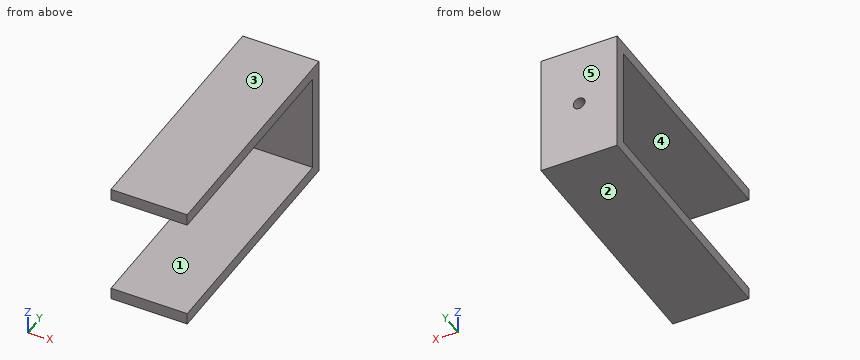
Autodesk Inventor part; units mm, degrees
ref_plane "YZ Plane" through (0, 0, 0) normal (1, 0, 0) x (0, 1, 0)
ref_plane "XZ Plane" through (0, 0, 0) normal (0, 1, 0) x (-1, 0, 0)
ref_plane "XY Plane" through (0, 0, 0) normal (0, 0, 1) x (1, 0, 0)
sketch "Boceto1" plane through (0, 0, 0) normal (0, 0, 1) x (1, 0, 0)
  line L0 (0, 0) -> (130, 0)
  line L1 (130, 0) -> (130, 420)
  line L2 (130, 420) -> (0, 420)
  line L3 (0, 420) -> (0, 0)
  circle A0 centre (65, 210) radius 10
  dimension "d0" = 130
  dimension "d1" = 420
  dimension "d2" = 130
  dimension "d10" = 20
extrude "Extrusión1" add sketch "Boceto1" along normal blind 210 contours L3 L2 L1 L0 | A0
sketch "Boceto2" plane through (130, 0, 0) normal (1, 0, 0) x (0, 0, -1)
  line L0 (-210, 420) -> (-210, 0)
  line L1 (-210, 0) -> (-190, 0)
  line L2 (0, 0) -> (-210, 0)
  line L3 (-190, 0) -> (-190, 400)
  line L4 (-190, 400) -> (-20, 400)
  line L5 (0, 420) -> (0, 0)
  line L6 (-20, 400) -> (-20, 0)
  line L7 (-20, 0) -> (0, 0)
  dimension "d5" = 20
  dimension "d6" = 400
  dimension "d7" = 170
extrude "Extrusión2" cut sketch "Boceto2" against normal blind 210
sketch "Boceto3" plane through (0, 420, 0) normal (0, 1, 0) x (1, 0, 0)
  line L0 (130, 0) -> (0, 0)
  line L1 (130, -210) -> (0, -210)
  line L2 (0, 0) -> (130, -210)
  line L3 (130, 0) -> (0, -210)
  circle A0 centre (65, -105) radius 10
  dimension "d11" = 20
hole "Agujero1" at (65, 420, 105) direction (0, -1, 0) diameter 20 end through all
properties part number "Soporteguia"
The listing builds one solid part. Answer for the finished solid, in the listing's coordinates (mm). Face numbers are marked on the shaded views. A direction names the side the tool comes from. Coordinates: 2 decimals unless noted, no trailing zeros. Loops run counter-clockwise (first coordinate to the right, second up) from the corner with the lowest first, then second, coordinate; pieces in that order, holes last. Notation, with made-up numbers: M -38,62 L -1,62 A32 ccw -1,100 Z; hole C 59.25,-24 d9. An arc over 180 degrees is marked long. Answer as a JSON object with one key per item and string values. Group by question number.
Item 1: Consider L1, parallel to Z at x = 82, y = 118; L2, parallel to X at y = 408.75, z = 105; L3, parallel to Z at x = 65, y = 414. Determine where each line is inside the solid, lowest interval first.
Item 2: Which of the six approach directions +Z, -Z, +X, -X, +Y, -Y give full straight-line access (tool end or side, diameter ignored) to the marked faces 4 and 5?
Item 3: Section D-D (x = 92.5) is taken. Write down the section's boundary in (y, z).
Item 4: This flat-tipped pin is pushed along its axis until it touches: P1, Ø2, axis at x = 111, z = 53.5, coming from the -Y side. Where does it stop, or does it pass through?
Item 5: Section B-B (x = 65) is taken. Write down the section's boundary in (y, z).
Item 6: Determine the mould class of the marked faces 1, 2 and 3 for opening direction Z: +Z half, -Z half, draft (parallel to the pull), parting line (faces both ways), or undercut.
Item 7: Section A-A (z = 105) is taken. Write down the section's boundary in (x, y), and give its area (3 significant figures).
Item 8: Section C-C (y = 245) is taken. Write down the section's boundary in (x, z).
Solved:
{
 "1": {"L1": "z = 0 to 20, 190 to 210", "L2": "x = 0 to 55, 75 to 130", "L3": "z = 0 to 95, 115 to 210"},
 "2": {"face 4": "+X, -X, -Y", "face 5": "+Z, -Z, +X, -X, +Y"},
 "3": {"outline": "M 0,0 L 420,0 L 420,210 L 0,210 L 0,190 L 400,190 L 400,20 L 0,20 Z"},
 "4": {"P1": "stops at y = 400"},
 "5": {"outline": "M 0,0 L 420,0 L 420,95 L 400,95 L 400,20 L 0,20 Z; M 0,190 L 400,190 L 400,115 L 420,115 L 420,210 L 0,210 Z"},
 "6": {"face 1": "undercut", "face 2": "-Z half", "face 3": "+Z half"},
 "7": {"outline": "M 0,400 L 55,400 L 55,420 L 0,420 Z; M 75,400 L 130,400 L 130,420 L 75,420 Z", "area": "2,200 mm2"},
 "8": {"outline": "M 0,0 L 130,0 L 130,20 L 0,20 Z; M 0,190 L 130,190 L 130,210 L 0,210 Z"}
}
